Design review of the part built by this model. Coordinates are the model's own, in mm. Face numbers are marked on the shaded views. A direction names the side the tool comes from. Round coordinates to 2 decimals unless told otherwise and drop trailing zeros. Loops run counter-clockwise (first coordinate to the right, second up) from the corner with the lowest first, then second, coordinate; pieces in that order, holes last. Notation, with made-up numbers: M -18.5,-27.5 L 28.5,-27.5 A34 cw 28.5,11.5 Z; hole C 45.25,22.5 d11. An arc over 180 degrees is marked long. One line per item, written item: value. Start each with the question number.
Item 1: We need section C-C (y = 20.5). Write out the cut boundary in (x, z), then the cut area to 3 significant figures.
Item 2: Mouldability with a two-part tool opening along Z and no side actions: class the marked faces 1, 2 and 3 as released by +Z, released by -Z, zero draft, split by the parting line, or undercut.
Item 3: For line 1 along X through (y, z) = (1, 15.5); line 2 along Y through (x, z) = (-3, 15); line 3 along X through (y, z) = (-2, -14), list the stretches that pass through material, from the lowest coordinate up.
Item 4: For the marked faces 4 and 5, list the 3-axis set-ups (+Z, -Z, +X, -X, +Y, -Y) from which the entire face can be reached by the end or side of a thin tool; tool diameter is ignored.
Item 5: We need section D-D (z = -15.5). Write out the cut boundary in (x, y).
Item 6: We need section A-A (y = 1). Write out the cut boundary in (x, z), then the cut area to 3 significant figures.
Item 7: Clearance check with flat-ended pins moving along their axes: pin 1 (2 mm diameter, centred on x = 41.5, z = -15, fed in from -Y) (3 decimals); pin 2 (1.5 mm diameter, centred on x = 89, z = 6.5, fed in from -Y); pin 3 (10 mm diameter, centred on y = 11.5, z = 7, fed in from -X). State where each tip first meets the part, or that it passes through.
Item 8: We need section B-B (x = -3.36). Write out the cut boundary in (y, z), then the cut area to 3 significant figures.
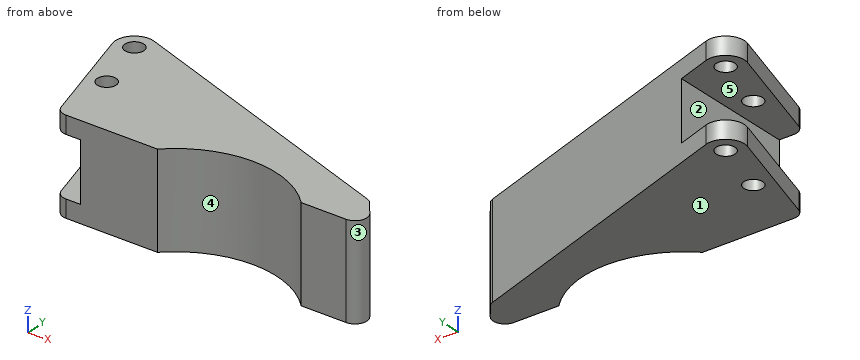
from build123d import *

# Parameters (mm, degrees)
SKETCH1_R               = 4
BOSS_EXTRUDE1_DEPTH     = 20
CUT_EXTRUDE1_DEPTH      = 138.969985504
CUT_EXTRUDE1_DEPTH_BACK = 138.969985504
SKETCH3_W               = 25
SKETCH3_H               = 25


with BuildPart() as part:
    # Sketch1 → Boss-Extrude1 (new, symmetric)
    with BuildSketch(Plane.XY):
        with BuildLine():
            Line((0, -5), (39.194156399, -5))
            ThreePointArc((39.194156399, -5), (70, 8), (100.805843601, -5))
            Line((100.805843601, -5), (120, -5))
            ThreePointArc((120, -5), (124.494057443, -2.191676915), (123.939808781, 3.07862092))
            Line((123.939808781, 3.07862092), (119.251326027, 9.07862092))
            ThreePointArc((119.251326027, 9.07862092), (118.224409903, 10.063872091), (116.961517246, 10.71990466))
            Line((116.961517246, 10.71990466), (-8.05, 54.421847456))
            ThreePointArc((-8.05, 54.421847456), (-16.204790321, 52.665436802), (-18.363488412, 44.607794087))
            Line((-18.363488412, 44.607794087), (-4.795930257, -1.413878695))
            ThreePointArc((-4.795930257, -1.413878695), (-2.994211626, -4.004334744), (0, -5))
        make_face()
        with Locations((-3.36, 22)):
            Circle(SKETCH1_R, mode=Mode.SUBTRACT)
        with Locations((-10.69, 46.87)):
            Circle(SKETCH1_R, mode=Mode.SUBTRACT)
    extrude(amount=BOSS_EXTRUDE1_DEPTH, both=True)

    # Sketch3 → Cut-Extrude1 (cut, two sides: drawn at the far end of the back side and taken through both)
    with BuildSketch(Plane(origin=(0, 0, 0), x_dir=(1, 0, 0), z_dir=(0, 1, 0)).offset(-CUT_EXTRUDE1_DEPTH_BACK)):
        with Locations((-6.19, 0)):
            Rectangle(SKETCH3_W, SKETCH3_H)
    extrude(amount=CUT_EXTRUDE1_DEPTH + CUT_EXTRUDE1_DEPTH_BACK, mode=Mode.SUBTRACT)


solid = part.part
A:
1. outline: M -11.26,-20 L -7.07,-20 L -7.07,-12.5 L -11.26,-12.5 Z; M -11.26,12.5 L -7.07,12.5 L -7.07,20 L -11.26,20 Z; M 0.35,-20 L 88.99,-20 L 88.99,20 L 0.35,20 L 0.35,12.5 L 6.31,12.5 L 6.31,-12.5 L 0.35,-12.5 Z
1. area: 3,460 mm2
2. face 1: released by -Z
2. face 2: undercut
2. face 3: zero draft
3. line 1: -5.51 to 46.48, 93.52 to 124.9
3. line 2: -4 to 18.02, 25.98 to 52.66
3. line 3: -4.58 to 42.43, 97.57 to 124.58
4. face 4: +Z, -Z, -Y
4. face 5: -X, +Y, -Y
5. outline: M -18.36,44.61 L -4.8,-1.41 A5 ccw 0,-5 L 39.19,-5 A43 cw 100.81,-5 L 120,-5 A5 ccw 123.94,3.08 L 119.25,9.08 A5 ccw 116.96,10.72 L -8.05,54.42 A8 ccw Z; hole C -10.69,46.87 d8; hole C -3.36,22 d8
6. outline: M -5.51,-20 L 46.48,-20 L 46.48,20 L -5.51,20 L -5.51,12.5 L 6.31,12.5 L 6.31,-12.5 L -5.51,-12.5 Z; M 93.52,-20 L 124.9,-20 L 124.9,20 L 93.52,20 Z
6. area: 3,040 mm2
7. pin 1: y = -3.715
7. pin 2: y = 3.2
7. pin 3: x = 6.31
8. outline: M -3.7,-20 L 18,-20 L 18,-12.5 L -3.7,-12.5 Z; M -3.7,12.5 L 18,12.5 L 18,20 L -3.7,20 Z; M 26,-20 L 52.78,-20 L 52.78,-12.5 L 26,-12.5 Z; M 26,12.5 L 52.78,12.5 L 52.78,20 L 26,20 Z
8. area: 727 mm2
